from build123d import *

# Parameters (mm, degrees)
SKETCH_R        = 7.5
SKETCH_R_2      = 4
PAD_DEPTH       = 24
CHAMFER_SIZE    = 1
CHAMFER001_SIZE = 1


with BuildPart() as part:
    # Sketch → Pad (new body)
    with BuildSketch(Plane.XY):
        Circle(SKETCH_R)
        Circle(SKETCH_R_2, mode=Mode.SUBTRACT)
    extrude(amount=PAD_DEPTH)

    # Chamfer
    chamfer_edges = [part.edges().sort_by_distance(p)[0] for p in [
        (-7.5, 0, 24),
    ]]
    chamfer(chamfer_edges, length=CHAMFER_SIZE)

    # Chamfer001
    chamfer001_edges = [part.edges().sort_by_distance(p)[0] for p in [
        (-7.5, 0, 0),
    ]]
    chamfer(chamfer001_edges, length=CHAMFER001_SIZE)


solid = part.part
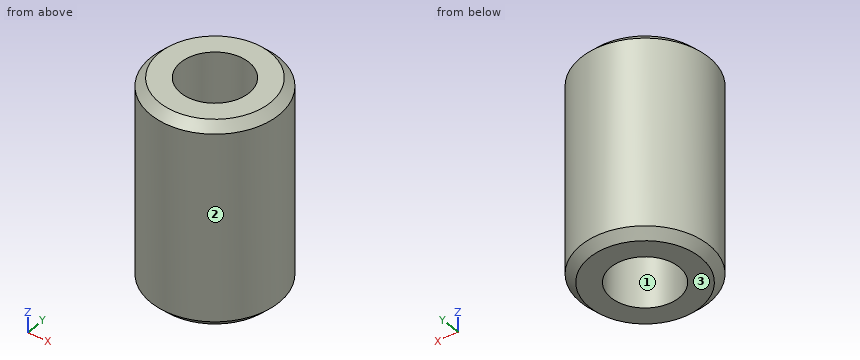
The listing builds one solid part. Answer for the finished solid, in the listing's coordinates (mm). Face numbers are marked on the shaded views. Give positions to 0.01 mm unless a question says otherwise; leave off trailing zeros. Order: outer loops, then holes, each group sorted by start corner. A loop starts at its lowest first (then second) coordinate and runs counter-clockwise, first axis right, second up. Notation, with made-up numbers: (74, -37) - (94, -37) arc R26 cw to (94, 0) - close; hole circle Ø4 at (77.5, -0.5). An arc over 180 degrees is marked (long way). Use one line per item in the form item = value.
1) The mould has two halves that part along Y. Classify the marked faces 1, 2 and 3: released by +Y, released by -Y, zero draft, split by the parting line, or undercut.
Verdict:
face_1 = undercut
face_2 = split by the parting line
face_3 = zero draft
2) Each of these flat-tipped pins is pushed along its axis until it touches: pin 1 (2 mm diameter, centred on x = -5, z = 14.5, fed in from -Y); pin 2 (3 mm diameter, centred on x = -3.5, z = 9.5, fed in from -Y); pin 3 (3 mm diameter, centred on x = 4.5, z = 18.5, fed in from +Y). Where does it stop, or does it pass through?
Verdict:
pin_1 = -6.34
pin_2 = -7.23
pin_3 = 6.87
3) Find section A-A on x = 0. Determine the outline of the cut face in (y, z).
Verdict:
outline = (-7.5, 1) - (-6.5, 0) - (-4, 0) - (-4, 24) - (-6.5, 24) - (-7.5, 23) - close; (4, 0) - (6.5, 0) - (7.5, 1) - (7.5, 23) - (6.5, 24) - (4, 24) - close
4) Find section C-C on z = 15.5. Determine the outline of the cut face in (x, y).
Verdict:
outline = circle Ø15 at (0, 0); hole circle Ø8 at (0, 0)
5) Consider probe 1 along Y at (x, z) = (0, 13.75); probe 2 along Y at (x, z) = (-3, 15); probe 3 along X at (y, z) = (-2.25, 10.25). Determine where each line is inside the solid, lowest interval first. Write a range as [from, to].
Verdict:
probe_1 = [-7.5, -4], [4, 7.5]
probe_2 = [-6.87, -2.65], [2.65, 6.87]
probe_3 = [-7.15, -3.31], [3.31, 7.15]
